Geometry check sheet. Reference: the model listing, model coordinates, mm. A direction names the side the tool comes from. Coordinates: 2 decimals unless noted, no trailing zeros. Order: outer loops, then holes, each group sorted by start corner. A loop starts at its lowest first (then second) coordinate and runs counter-clockwise, first axis right, second up. Notation, with made-up numbers: (6, 55) - (13, 55) arc R16 ccw to (13, 59) - close; hole circle Ø2 at (-5.5, 31.5). An arc over 180 degrees is marked (long way). Use CSV: the item, a comma, the result in double quotes. Start each with the question number.
1) Sectioned sample at A-A, the plane y = 29. Record the cut outline in (x, z).
2) Sectioned sample at D-D, the plane z = 46. Record the cut outline in (x, y).
3) Sectioned sample at C-C, the plane z = -14. Record the cut outline in (x, y).
4) Depth check by flat-ended pin: P1, Ø2, axis at y = -28, z = 20.5, coming from the +X side; P2, Ø12, axis at y = 41, z = -16, coming from the -X side; P3, Ø12, axis at x = -162, z = -31.5, coming from the +Y side. Enter the tip coordinate at first touch or a pass-through.
5) Tool access check on faces 1 (the flat face through (93.388, -1, 22)), 2 (the flat face through (-13, 63.5, 16)). Record the directions out of +Z, -Z, +X, -X, +Y, -Y that give a thin tool (end or side, any length) a straight path to the whole face; none if there is none.
6) Thickness scan on probe 1 along Y at (x, z) = (-54, 29); probe 2 along X at (y, z) = (2, -28); probe 3 along Y at (x, z) = (45, 40.5). Record the ranges inside material, lowest first. Write a range as [from, to].
from build123d import *

# Parameters (mm, degrees)
F0_W         = 254
F0_H         = 76.2
F1_DEPTH     = 63.5
F2_SIZE      = 63.49999
F3_DEPTH     = 63.5
F4_T1_DEPTH  = 463.9752430668
F5_T1_DEPTH  = 463.9752430668
F6_DEPTH     = 63.5
F7_T1_DEPTH  = 418.1847418685
F0_H_2       = 50.8
F8_DEPTH     = 63.5
F9_SIZE      = 38.1
F10_DEPTH    = 63.5
F11_T1_DEPTH = 463.7665363346


# Not quite as in the source:
# - a fillet or chamfer that OpenCascade refuses, or shapes differently, is made with other operations: its cross-section is extruded or revolved along the edge and cut away or added
# - a fillet or chamfer is up to 0.001 mm smaller than in the source, because OpenCascade refuses the exact size


with BuildPart() as f1:
    # F0 (on Front) → F1 (new body, symmetric)
    with BuildSketch(Plane.XZ):
        with Locations((-33.6120952994, -22.0760072346)):
            Rectangle(F0_W, F0_H)
    extrude(amount=F1_DEPTH, both=True)

    # F2 (size 63.5 in the source; OpenCascade refuses exactly that, so slightly less here)
    f2_edges = [f1.edges().sort_by_distance(p)[0] for p in [
        (-33.612095, -63.5, -60.176007),
        (-33.612095, 63.5, -60.176007),
    ]]
    chamfer(f2_edges, length=F2_SIZE)

    # F0 (on Front) → F3 (join, symmetric)
    with BuildSketch(Plane.XZ):
        Polygon((207.6879047006, 16.0239927654), (93.3879047006, 16.0239927654), (93.3879047006, -60.1760072346), align=None)
    extrude(amount=F3_DEPTH, both=True)

    # F4: chamfer of 63.5 on 1 edges, made by hand

    # F4_s2 → F4_t1 (cut)
    with BuildSketch(Plane(origin=(-98.9957457875, 0, -65.9971638583), x_dir=(0, 1, 0), z_dir=(0.8320502943, 0, 0.5547001962))):
        Polygon((-63.5, -38.3717535941), (0, -101.8717535941), (-63.5, -101.8717535941), align=None)
    extrude(amount=F4_T1_DEPTH, mode=Mode.SUBTRACT)

    # F5: chamfer of 63.5 on 1 edges, made by hand

    # F5_s2 → F5_t1 (cut)
    with BuildSketch(Plane(origin=(-98.9957457875, 0, -65.9971638583), x_dir=(0, 1, 0), z_dir=(0.8320502943, 0, 0.5547001962))):
        Polygon((63.5, -38.3717535941), (0, -101.8717535941), (63.5, -101.8717535941), align=None)
    extrude(amount=F5_T1_DEPTH, mode=Mode.SUBTRACT)

    # F0 (on Front) → F6 (join, symmetric)
    with BuildSketch(Plane.XZ):
        Polygon((-160.6120952994, -60.1760072346), (-160.6120952994, 16.0239927654), (-211.4120952994, 16.0239927654), align=None)
    extrude(amount=F6_DEPTH, both=True)

    # F7: chamfer of 63.5 on 2 edges, made by hand

    # F7_s2 → F7_t1 (cut)
    with BuildSketch(Plane(origin=(-163.0291436318, 0, 244.5437154477), x_dir=(0, 1, 0), z_dir=(0.5547001962, 0, -0.8320502943))):
        Polygon((63.5, -103.5169841892), (0, -167.0169841892), (63.5, -167.0169841892), align=None)
        Polygon((-63.5, -103.5169841892), (0, -167.0169841892), (-63.5, -167.0169841892), align=None)
    extrude(amount=F7_T1_DEPTH, mode=Mode.SUBTRACT)

    # F0 (on Front) → F8 (join, symmetric)
    with BuildSketch(Plane.XZ):
        with Locations((-33.6120952994, 41.4239927654)):
            Rectangle(F0_W, F0_H_2)
    extrude(amount=F8_DEPTH, both=True)

    # F9
    f9_edges = [f1.edges().sort_by_distance(p)[0] for p in [
        (-33.612095, -63.5, 66.823993),
        (-33.612095, 63.5, 66.823993),
        (93.387905, 0, 66.823993),
    ]]
    chamfer(f9_edges, length=F9_SIZE)

    # F0 (on Front) → F10 (join, symmetric)
    with BuildSketch(Plane.XZ):
        Polygon((-211.4120952994, 16.0239927654), (-160.6120952994, 16.0239927654), (-160.6120952994, 66.8239927654), align=None)
    extrude(amount=F10_DEPTH, both=True)

    # F11: chamfer of 76.2 on 2 edges, made by hand

    # F11_s2 → F11_t1 (cut)
    with BuildSketch(Plane(origin=(91.6721800978, 0, 91.6721800978), x_dir=(0, 1, 0), z_dir=(-0.7071067812, 0, -0.7071067812))):
        Polygon((-63.5, -84.6216001572), (12.7, -160.8216001572), (-63.5, -160.8216001572), align=None)
        Polygon((63.5, -84.6216001572), (-12.7, -160.8216001572), (63.5, -160.8216001572), align=None)
    extrude(amount=F11_T1_DEPTH, mode=Mode.SUBTRACT)


solid = f1.part
Evaluation:
1,outline,"(-166.91, 1.55) - (-145.09, -31.18) - (84.61, -31.18) - (155.41, 16.02) - (93.39, 16.02) - (93.39, 28.72) - (58.89, 63.22) - (-105.24, 63.22) - close"
2,outline,"(-163.48, 0) - (-98.1, -46.22) - (76.11, -46.22) - (76.11, 46.22) - (-98.1, 46.22) - close"
3,outline,"(-191.4, 0) - (-135.9, -46.18) - (79.41, -46.18) - (162.65, 0) - (79.41, 46.18) - (-135.9, 46.18) - close"
4,P1,"x = 93.39"
4,P2,"x = -149.03"
4,P3,"y = 20.75"
5,face 1,"+Z, +X, +Y, -Y"
5,face 2,"+Z, -Z, +X, -X, +Y"
6,probe 1,"[-63.22, 63.22]"
6,probe 2,"[-179.66, 138.05]"
6,probe 3,"[-51.72, 51.72]"
